The model under review builds one solid part; all positions refer to its coordinate system, in mm. Give positions to 0.01 mm unless a question says otherwise; leave off trailing zeros. Order: outer loops, then holes, each group sorted by start corner. A loop starts at its lowest first (then second) coordinate and runs counter-clockwise, first axis right, second up. Notation, with made-up numbers: (7.5, -29.75) - (23.5, -29.75) arc R19 ccw to (23.5, 7.25) - close; hole circle Ø8 at (-25, 80). An arc over 180 degrees is marked (long way). Use CSV: the item, a comma, the result in double quotes. Start each with the question number.
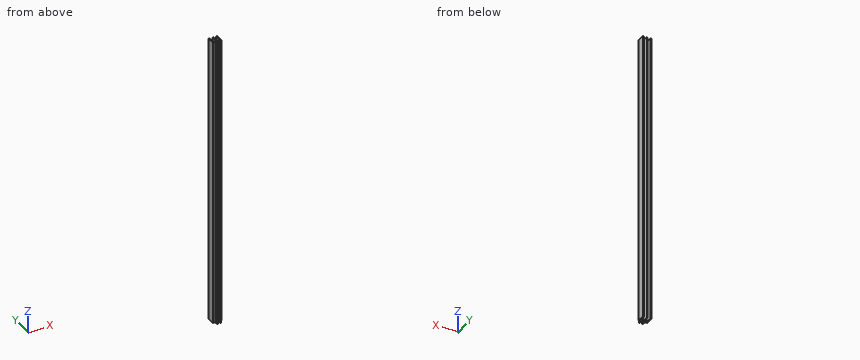
```python
from build123d import *

# Parameters (mm, degrees)
BOSS_EXTRU_1_DEPTH = 668


with BuildPart() as part:
    # Esquisse1 → Boss.-Extru.1 (new body)
    with BuildSketch(Plane.XY.offset(50)):
        Polygon((-1, 2.5), (-7.5, 2.5), (-7.5, 17.999999998), (-10, 17.999999998), (-10, 0), (-4, 0), (-4, -4.5), (-5, -4.5), (-3.75, -8), (-3, -8), (-3, 0), (3, 0), (3, -8), (3.75, -8), (5, -4.5), (4, -4.5), (4, 0), (10, 0), (10, 17.999999998), (7.5, 17.999999998), (7.5, 2.5), (1, 2.5), (1, 17.999999998), (-1, 17.999999998), align=None)
    extrude(amount=-BOSS_EXTRU_1_DEPTH)


solid = part.part
```
1. Consider section A-A (y = 13.5). Give the boundary of the cut face in (x, z).
2. To check wall thickness, follow L1, parallel to X at y = 5, z = -422.5; L2, parallel to X at y = -0.5, z = -99.5; L3, parallel to Y at x = 2.5, z = -154. State the ranges of each line that lie inside material, in increasing order. Write a range as [from, to].
3. Clearance check with flat-ended pins moving along their axes: pin 1 (2 mm diameter, centred on x = 5.5, z = -387, fed in from +Y); pin 2 (4 mm diameter, centred on y = -3, z = -330, fed in from +X); pin 3 (3.5 mm diameter, centred on y = -3.5, z = -212.5, fed in from -X); pin 4 (1.5 mm diameter, centred on x = -2.5, y = 9.5, fed in from +Z). State where each tip first meets the part, or that it passes through.
4. Consider section B-B (z = -365.5). Give the boundary of the cut face in (x, y).
Answers follow:
1,outline,"(-10, -618) - (-7.5, -618) - (-7.5, 50) - (-10, 50) - close; (-1, -618) - (1, -618) - (1, 50) - (-1, 50) - close; (7.5, -618) - (10, -618) - (10, 50) - (7.5, 50) - close"
2,L1,"x = [-10, -7.5], [-1, 1], [7.5, 10]"
2,L2,"x = [-4, -3], [3, 4]"
2,L3,"y = [0, 2.5]"
3,pin 1,"stops at y = 2.5"
3,pin 2,"stops at x = 5"
3,pin 3,"stops at x = -5"
3,pin 4,"passes through"
4,outline,"(-10, 0) - (-4, 0) - (-4, -4.5) - (-5, -4.5) - (-3.75, -8) - (-3, -8) - (-3, 0) - (3, 0) - (3, -8) - (3.75, -8) - (5, -4.5) - (4, -4.5) - (4, 0) - (10, 0) - (10, 18) - (7.5, 18) - (7.5, 2.5) - (1, 2.5) - (1, 18) - (-1, 18) - (-1, 2.5) - (-7.5, 2.5) - (-7.5, 18) - (-10, 18) - close"
